Could you check a few things on this drawing? It's one solid part, dimensions in mm from its lowest x, y, z. A direction names the side the tool comes from. Coordinates: 2 decimals unless noted, no trailing zeros. Write each loop counter-clockwise with the first axis right and the second up, starting at its lowest first coordinate (ties: lowest second). Pieces come first, ordered by that corner, then holes. Notation, with made-up numbers: (5.5, 43.5) - (30.5, 43.5) arc R23 ccw to (30.5, 74.5) - close; hole circle Ø2 at (-39, -17). An arc over 180 degrees is marked (long way). Answer as a JSON object with one key per item and string values. Group by question number.
1) If we section it at A-A (x = 40.5): Write out the boundary of the cut face in (y, z), plus the area to 3 significant figures.
2) Please list where these lines run through material, in increasing order: line 1 along Z through (x, y) = (89, 28); line 2 along Y through (x, z) = (75, 46); line 3 along Y through (x, z) = (41, 59.5).
3) If we section it at D-D (x = 89): Write out the boundary of the cut face in (y, z).
4) If we section it at B-B (y = 15): Write out the boundary of the cut face in (x, z).
5) If we section it at C-C (z = 31): Write out the boundary of the cut face in (x, y).
6) On a 3-axis mill with a long thin cutter (end or side, diameter ignored), from which of +Z, -Z, +X, -X, +Y, -Y can I reach the whole of each face in a straight line? I mean the marked faces 1 and 2. Say none if no direction works.
7) Will these pins go through, and if not, where does the flat tip stop? pin 1 Ø4 at (x, z) = (37.4, 15.6) entering from +Y; pin 2 Ø1 at (x, z) = (38, 51.5) entering from -Y; pin 3 Ø6 at (x, y) = (34.84, 20.66) entering from -Z; pin 4 Ø2.5 at (x, y) = (46.16, 9.34) entering from -Z.
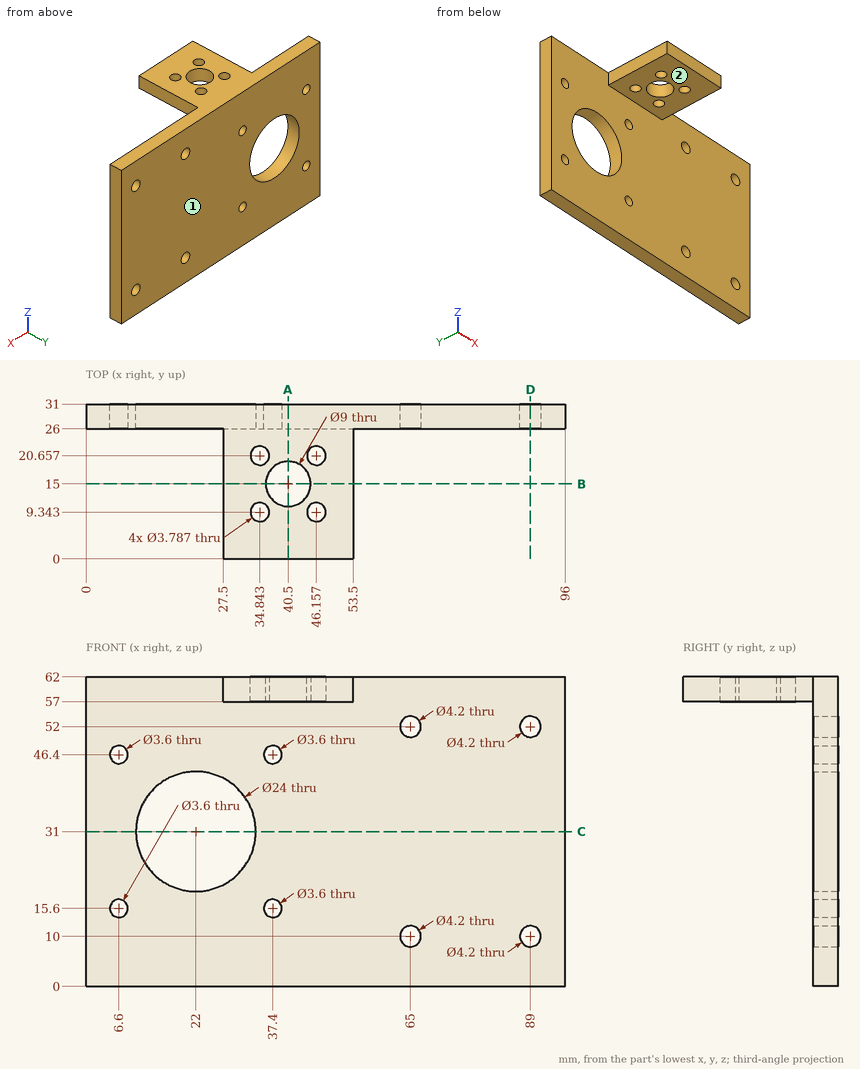
Here are the results:
{
 "1": {"outline": "(0, 57) - (10.5, 57) - (10.5, 62) - (0, 62) - close; (19.5, 57) - (26, 57) - (26, 0) - (31, 0) - (31, 62) - (19.5, 62) - close", "area": "395 mm²"},
 "2": {"line 1": "z = 0 to 7.9, 12.1 to 49.9, 54.1 to 62", "line 2": "y = 26 to 31", "line 3": "y = 0 to 10.53, 19.47 to 31"},
 "3": {"outline": "(26, 0) - (31, 0) - (31, 7.9) - (26, 7.9) - close; (26, 12.1) - (31, 12.1) - (31, 49.9) - (26, 49.9) - close; (26, 54.1) - (31, 54.1) - (31, 62) - (26, 62) - close"},
 "4": {"outline": "(27.5, 57) - (36, 57) - (36, 62) - (27.5, 62) - close; (45, 57) - (53.5, 57) - (53.5, 62) - (45, 62) - close"},
 "5": {"outline": "(0, 26) - (10, 26) - (10, 31) - (0, 31) - close; (34, 26) - (96, 26) - (96, 31) - (34, 31) - close"},
 "6": {"face 1": "+Z, -Z, +X, -X, +Y", "face 2": "-Z, +X, -X, -Y"},
 "7": {"pin 1": "stops at y = 31", "pin 2": "stops at y = 26", "pin 3": "stops at z = 57", "pin 4": "passes through"}
}
